Autodesk Inventor part; units mm, degrees
ref_plane "YZ Plane" through (0, 0, 0) normal (1, 0, 0) x (0, 1, 0)
ref_plane "XZ Plane" through (0, 0, 0) normal (0, 1, 0) x (-1, 0, 0)
ref_plane "XY Plane" through (0, 0, 0) normal (0, 0, 1) x (1, 0, 0)
sketch "Sketch1" plane through (0, 0, 0) normal (0, 0, 1) x (1, 0, 0)
  circle A0 centre (0, 0) radius 15.875
  circle A1 centre (0, 0) radius 25.4
  dimension "d0" = 31.75
  dimension "d1" = 50.8
extrude "Extrusion1" add sketch "Sketch1" along normal blind 8.89
chamfer "Chamfer1" distance 0.7937 angle 45 1 edges at (-25.4, 0, 0)
chamfer "Chamfer2" distance 3.175 angle 45 2 edges at (-15.875, 0, 8.89) (-15.875, 0, 0)
properties part number "Tire" material "Rubber, Silicone"
Check sheet for the modelled part. Datum: model origin and axes. Units: mm. Coordinates: 2 decimals unless noted, no trailing zeros. Loops run counter-clockwise (first coordinate to the right, second up) from the corner with the lowest first, then second, coordinate; pieces in that order, holes last. Notation, with made-up numbers: (51, 72.5) -> (110, 72.5) arc R32 ccw to (110, 109.5) -> close; hole circle Ø10 at (-9.75, 34.25). An arc over 180 degrees is marked (long way). Write item = value, one per line. Start each with the question number.
1. Depth check by flat-ended pin: P1, Ø3, axis at y = 11.5, z = 1.5, coming from the +X side; P2, Ø2, axis at x = -7.5, z = 5, coming from the -Y side. Enter the tip coordinate at first touch or a pass-through.
2. Draft check along Y on faces 1 (the cylindrical face through (-3.441, 15.497, 4.427)), 2 (the conical face through (-16.058, -0.707, 2.976)), 3 (the flat face through (4, 19, 8.89)), 4 (the cylindrical face through (-5.506, 24.796, 4.785)). Enter one of: released by +Y, released by -Y, zero draft, split by the parting line, or undercut.
3. Section check D-D on z = 7.5. Record the cut outline in (x, y), then the cut area to 3 significant figures.
4. Section check C-C on z = 1.5. Record the cut outline in (x, y).
5. Section check A-A on x = 0. Record the cut outline in (y, z) (3 decimals).
6. Material ranges on line 1 (Y direction, x = 0, z = 5.1) (3 decimals); line 2 (Y direction, x = -2, z = 4.25); line 3 (X direction, y = -11.5, z = 6), recorded low to high.
Responses:
q1.P1 = 23.35
q1.P2 = -24.55
q2.face_1 = undercut
q2.face_2 = undercut
q2.face_3 = zero draft
q2.face_4 = split by the parting line
q3.outline = circle Ø50.8 at (0, 0); hole circle Ø35.32 at (0, 0)
q3.area = 1,050 mm2
q4.outline = circle Ø50.8 at (0, 0); hole circle Ø35.1 at (0, 0)
q5.outline = (-25.4, 0.794) -> (-24.606, 0) -> (-19.05, 0) -> (-15.875, 3.175) -> (-15.875, 5.715) -> (-19.05, 8.89) -> (-25.4, 8.89) -> close; (15.875, 3.175) -> (19.05, 0) -> (24.606, 0) -> (25.4, 0.794) -> (25.4, 8.89) -> (19.05, 8.89) -> (15.875, 5.715) -> close
q6.line_1 = -25.4 to -15.875, 15.875 to 25.4
q6.line_2 = -25.32 to -15.75, 15.75 to 25.32
q6.line_3 = -22.65 to -11.35, 11.35 to 22.65
